from build123d import *

# Parameters (mm, degrees)
BOSS_EXTRUDE1_DEPTH      = 3
M3_CLEARANCE_HOLE1_D     = 3.2
M3_CLEARANCE_HOLE2_D     = 3.2
F_4_0_4_DIAMETER_HOLE1_D = 4
CUT_EXTRUDE3_DEPTH       = 3
FILLET5_R                = 3
M3_CLEARANCE_HOLE3_D     = 3.2
CUT_EXTRUDE4_START       = -3
CUT_EXTRUDE4_DEPTH       = 3
FILLET6_R                = 3


with BuildPart() as part:
    # Sketch2 → Boss-Extrude1 (new body)
    with BuildSketch(Plane(origin=(0, 0, 0), x_dir=(1, 0, 0), z_dir=(0, 1, 0))):
        with BuildLine():
            Line((-16.5, -13.85), (-42.5, -13.85))
            Line((-42.5, -13.85), (-42.5, 7.15))
            Line((-42.5, 7.15), (-24.825, 24.825))
            Line((-24.825, 24.825), (25.724873734, -25.724873734))
            Line((25.724873734, -25.724873734), (16.974873734, -34.474873734))
            ThreePointArc((16.974873734, -34.474873734), (14.482141695, -35.49995444), (12, -34.449489743))
            Line((12, -34.449489743), (12, -39))
            Line((12, -39), (-12, -39))
            Line((-12, -39), (-12, -34.449489743))
            ThreePointArc((-12, -34.449489743), (-17.17260394, -34.259908888), (-16.5, -29.127718677))
            Line((-16.5, -29.127718677), (-16.5, -13.85))
        make_face()
    extrude(amount=BOSS_EXTRUDE1_DEPTH)

    # Mirror5: part across plane


with BuildPart() as part_1:
    add(part.part)
    add(part.part.mirror(Plane(origin=(25.724873734, 3, 25.724873734), x_dir=(0.7071067811865465, 0, 0.7071067811865487), z_dir=(-0.7071067811865486, 0, 0.7071067811865465))))

    # M3 Clearance Hole1 (through all)
    with Locations(Plane(origin=(0, 3, 0), x_dir=(1, 0, 0), z_dir=(0, 1, 0))):
        with Locations((-39.5, 4.15), (-19.5, 4.15), (-19.5, -10.85), (-39.5, -10.85), (-4.15, 19.5), (-4.15, 39.5), (10.85, 39.5), (10.85, 19.5)):
            Hole(M3_CLEARANCE_HOLE1_D / 2)

    # M3 Clearance Hole2 (through all)
    with Locations(Plane(origin=(0, 3, 0), x_dir=(1, 0, 0), z_dir=(0, 1, 0))):
        with Locations((-2.329371406, 8.693332437), (6.363961031, 6.363961031), (8.693332437, -2.329371406), (2.329371406, -8.693332437), (-6.363961031, -6.363961031), (-8.693332437, 2.329371406)):
            Hole(M3_CLEARANCE_HOLE2_D / 2)

    # Ø4.0 (4) Diameter Hole1 (through all)
    with Locations(Plane(origin=(0, 3, 0), x_dir=(1, 0, 0), z_dir=(0, 1, 0))):
        with Locations((0, 0)):
            Hole(F_4_0_4_DIAMETER_HOLE1_D / 2)

    # Sketch13 → Cut-Extrude3 (cut)
    with BuildSketch(Plane(origin=(0, 3, 0), x_dir=(1, 0, 0), z_dir=(0, 1, 0))):
        with BuildLine():
            Line((-39.671572875, 7.15), (-21.333717444, 7.15))
            ThreePointArc((-21.333717444, 7.15), (-19.129970762, 11.844586048), (-15.909902577, 15.909902577))
            Line((-15.909902577, 15.909902577), (-23.410786438, 23.410786438))
            Line((-23.410786438, 23.410786438), (-39.671572875, 7.15))
        make_face()
    cut_extrude3 = extrude(amount=-CUT_EXTRUDE3_DEPTH, mode=Mode.SUBTRACT)

    # Mirror6: Cut-Extrude3 across plane
    add(cut_extrude3.mirror(Plane(origin=(0, -28.792883686, 0), x_dir=(0.7071067811865467, 0, 0.7071067811865482), z_dir=(-0.7071067811865482, 0, 0.7071067811865468))), mode=Mode.SUBTRACT)

    # Fillet5
    fillet5_edges = [part_1.edges().sort_by_distance(p)[0] for p in [
        (-21.333717444, 1.5, -7.15),
        (-39.671572875, 1.5, -7.15),
        (-7.15, 1.5, -21.333717444),
        (-7.15, 1.5, -39.671572875),
    ]]
    fillet(fillet5_edges, radius=FILLET5_R)

    # M3 Clearance Hole3 (through all)
    with Locations(Plane(origin=(0, 3, 0), x_dir=(1, 0, 0), z_dir=(0, 1, 0))):
        with Locations((-12.727922061, 12.727922061)):
            Hole(M3_CLEARANCE_HOLE3_D / 2)

    # Sketch16 → Cut-Extrude4 (cut)
    with BuildSketch(Plane(origin=(0, 3, 0), x_dir=(1, 0, 0), z_dir=(0, 1, 0)).offset(CUT_EXTRUDE4_START)):
        with BuildLine():
            Line((-16.5, -13.85), (-10.493288043, -8.808002387))
            ThreePointArc((-10.493288043, -8.808002387), (9.687362902, -9.687362902), (8.808002387, 10.493288043))
            Line((8.808002387, 10.493288043), (13.85, 16.5))
            Line((13.85, 16.5), (29.127718677, 16.5))
            ThreePointArc((29.127718677, 16.5), (34.259908888, 17.17260394), (34.449489743, 12))
            Line((34.449489743, 12), (39, 12))
            Line((39, 12), (39, -12))
            Line((39, -12), (34.449489743, -12))
            ThreePointArc((34.449489743, -12), (35.49995444, -14.482141695), (34.474873734, -16.974873734))
            Line((34.474873734, -16.974873734), (16.974873734, -34.474873734))
            ThreePointArc((16.974873734, -34.474873734), (14.482141695, -35.49995444), (12, -34.449489743))
            Line((12, -34.449489743), (12, -39))
            Line((12, -39), (-12, -39))
            Line((-12, -39), (-12, -34.449489743))
            ThreePointArc((-12, -34.449489743), (-17.17260394, -34.259908888), (-16.5, -29.127718677))
            Line((-16.5, -29.127718677), (-16.5, -13.85))
        make_face()
    extrude(amount=CUT_EXTRUDE4_DEPTH, mode=Mode.SUBTRACT)

    # Fillet6
    fillet6_edges = [part_1.edges().sort_by_distance(p)[0] for p in [
        (-16.5, 1.5, 13.85),
        (-42.5, 1.5, 13.85),
        (-42.5, 1.5, -7.15),
        (-10.493288043, 1.5, 8.808002387),
        (8.808002387, 1.5, -10.493288043),
        (-7.15, 1.5, -42.5),
        (13.85, 1.5, -42.5),
        (13.85, 1.5, -16.5),
    ]]
    fillet(fillet6_edges, radius=FILLET6_R)


solid = part_1.part
Can you work these out from the model? Positions are in its coordinate system, mm. A direction names the side the tool comes from. Give positions to 0.01 mm unless a question says otherwise; leave off trailing zeros. Loops run counter-clockwise (first coordinate to the right, second up) from the corner with the lowest first, then second, coordinate; pieces in that order, holes last. Notation, with made-up numbers: (58, -5.5) -> (117, -5.5) arc R32 ccw to (117, 29.5) -> close; hole circle Ø3 at (45, 53.25). An arc over 180 degrees is marked (long way). Write item = value, one per line.
1) I need wall thicknesses on L1, parallel to Z at x = 0, y = 1.95; L2, parallel to X at y = 1.1, z = -39; L3, parallel to Z at x = -4.15, y = 2.35. Which ranges of each line are inside material? Lowest first, please. Write a range as from..to.
Check result:
L1 = -42.5..-2, 2..13.7
L2 = -10.65..-5.67, -2.63..9.33, 12.37..13.85
L3 = -42.5..-41.1, -37.9..-21.1, -17.9..13.06
2) Suppose I cut it at A-A on z = -30. Write out the boundary of the cut face in (x, y), then the cut area to 3 significant figures.
Check result:
outline = (-19.65, 0) -> (-16.82, 0) -> (-16.82, 3) -> (-19.65, 3) -> close; (-7.15, 0) -> (13.85, 0) -> (13.85, 3) -> (-7.15, 3) -> close
area = 71.5 mm2
3) Will these pins go through, and if not, where does the flat tip stop? pin 1 (1.5 mm diameter, centred on y = 1, z = -30, fed in from -X); pin 2 (1.5 mm diameter, centred on y = 1.5, z = -18.5, fed in from -X).
Check result:
pin_1 = -20.4
pin_2 = -31.9
4) Suppose I cut it at C-C on x = -27.5. Write out the boundary of the cut face in (y, z), then the cut area to 3 significant figures.
Check result:
outline = (0, -22.15) -> (3, -22.15) -> (3, -19.32) -> (0, -19.32) -> close; (0, -7.15) -> (3, -7.15) -> (3, 13.85) -> (0, 13.85) -> close
area = 71.5 mm2
5) For faces 1 (the flat face through (-42.5, 1, 3)), 2 (the cylindrical face through (-16.552, 1.521, 13.664)), 3 (the flat face through (11.837, 1.479, -14.102)), 4 (the cylindrical face through (-9, 1.5, -35.2)), which set-ups out of +Z, -Z, +X, -X, +Y, -Y let a thin tool reach every point of the face, with its end or its side?
Check result:
face_1 = +Z, -Z, -X, +Y, -Y
face_2 = +Z, +Y, -Y
face_3 = +X, +Y, -Y
face_4 = +Y, -Y
6) Thinking about a two-plate mould opening in Z: for faces 5 (the flat face through (-28, 1, 13.85)), 6 (the cylindrical face through (9.86, 1.52, -10.69)), 7 (the flat face through (-8, 0, -8)), which applies, released by +Z, released by -Z, zero draft, split by the parting line, or undercut?
Check result:
face_5 = released by +Z
face_6 = undercut
face_7 = zero draft
7) Suppose I cut it at D-D on y = 0.85. Give the number of separate pieces and of enclosed holes in the cut face, then the cut area to 3 significant figures.
Check result:
separate_pieces = 1
enclosed_holes = 17
area = 1,930 mm2
8) Suppose I cut it at B-B on x = -19.5. Write out the boundary of the cut face in (y, z), then the cut area to 3 significant figures.
Check result:
outline = (0, -30.15) -> (3, -30.15) -> (3, -27.32) -> (0, -27.32) -> close; (0, -11.22) -> (3, -11.22) -> (3, -5.75) -> (0, -5.75) -> close; (0, -2.55) -> (3, -2.55) -> (3, 9.25) -> (0, 9.25) -> close; (0, 12.45) -> (3, 12.45) -> (3, 13.85) -> (0, 13.85) -> close
area = 64.5 mm2
